```python
from build123d import *

# Parameters (mm, degrees)
F0_R     = 25.4
F1_DEPTH = 152.4
F2_R     = 22.225
F3_DEPTH = 146.05
F4_DEPTH = 25.4


with BuildPart() as f1:
    # F0 (on Front) → F1 (new body)
    with BuildSketch(Plane.XZ):
        Circle(F0_R)
    extrude(amount=F1_DEPTH)

    # F2 (on face) → F3 (cut)
    with BuildSketch(Plane.XZ.offset(152.4)):
        with Locations((-1.2778061209, 2.3061255924)):
            Circle(F2_R)
    extrude(amount=-F3_DEPTH, mode=Mode.SUBTRACT)

    # F4 (add): faces of the model
    f4_faces = [f1.faces().sort_by_distance(p)[0] for p in [
        (-24.6815795103, -152.4, 0),
        (0, 0, 0),
    ]]
    extrude(f4_faces, amount=F4_DEPTH, dir=(0, -1, 0))


solid = f1.part
```
Here's how the part is built. I have some questions about the finished solid (model axes, mm). Round coordinates to 2 decimals unless told otherwise and drop trailing zeros. Loops run counter-clockwise (first coordinate to the right, second up) from the corner with the lowest first, then second, coordinate; pieces in that order, holes last.
1. Suppose I cut it at C-C, the plane y = -14. Please give me the cut outline in (x, z).
Answers:
outline: circle Ø50.8 at (0, 0)
2. Will these pins go through, and if not, where does the flat tip stop? pin 1 (6 mm diameter, centred on y = -110, z = 18, fed in from +X); pin 2 (6 mm diameter, centred on x = 8, y = -45.5, fed in from -Z); pin 3 (1 mm diameter, centred on y = -49, z = 16.5, fed in from -X).
Answers:
pin 1: stops at x = 20.5
pin 2: stops at z = -24.9
pin 3: stops at x = -19.73
3. If I drill on probe 1 along X at (y, z) = (-140, 1); probe 2 along Z at (x, y) = (-4, -147); probe 3 along Y at (x, z) = (5.5, -10), over which ranges is the centre line in solid material (lowest first)?
Answers:
probe 1: x = -25.38 to -23.46, 20.91 to 25.38
probe 2: z = -25.08 to -19.75, 24.36 to 25.08
probe 3: y = -25.4 to 0
4. Thinking about a two-plate mould opening in Z: for faces 1 (the face through (7, -177.8, -19)), 2 (the face through (-2, -25.4, 3)), 3 (the face through (-5.506, -87.655, -24.796)), which applies, released by +Z, released by -Z, zero draft, split by the parting line, or undercut?
Answers:
face 1: zero draft
face 2: undercut
face 3: split by the parting line
5. Suppose I cut it at B-B, the plane z = -16. Please give me the cut outline in (x, y), and give its area (3 significant figures).
Answers:
outline: (-19.73, -177.8) - (-13.88, -177.8) - (-13.88, -25.4) - (11.33, -25.4) - (11.33, -177.8) - (19.73, -177.8) - (19.73, 0) - (-19.73, 0) - close
area: 3,170 mm2
6. Suppose I cut it at A-A, the plane x = -13. Please give me the cut outline in (y, z), and give its area (3 significant figures).
Answers:
outline: (-177.8, -21.82) - (0, -21.82) - (0, 21.82) - (-177.8, 21.82) - (-177.8, 21.19) - (-25.4, 21.19) - (-25.4, -16.58) - (-177.8, -16.58) - close
area: 2,000 mm2
7. Suppose I cut it at D-D, the plane y = -149.5. Please give me the cut outline in (x, z) (3 decimals).
Answers:
outline: circle Ø50.8 at (0, 0); hole circle Ø44.45 at (-1.278, 2.306)
